from build123d import *

# Parameters (mm, degrees)
SKETCH1_R           = 19
BOSS_EXTRUDE1_DEPTH = 25
FILLET1_R           = 0.5
SKETCH3_R           = 1.55
CUT_EXTRUDE1_DEPTH  = 26.0000001
SKETCH4_R           = 6.58897104
CUT_EXTRUDE2_DEPTH  = 26.0000001
CIRPATTERN1_COUNT   = 4


with BuildPart() as part:
    # Sketch1 → Boss-Extrude1 (new body)
    with BuildSketch(Plane.XY):
        Circle(SKETCH1_R)
    extrude(amount=BOSS_EXTRUDE1_DEPTH)

    # Sketch2 → Cut-Revolve1 (revolve, cut)
    with BuildSketch(Plane(origin=(0, 0, 0), x_dir=(0, 0, -1), z_dir=(1, 0, 0))):
        with BuildLine():
            Line((-24, 19), (-21.5, 19))
            ThreePointArc((-21.5, 19), (-22.75, 18.5), (-24, 19))
        make_face()
        with BuildLine():
            Line((-3.5, 19), (-1, 19))
            ThreePointArc((-1, 19), (-2.25, 18.7), (-3.5, 19))
        make_face()
    revolve(axis=Axis((0, 0, 8.4), (0, 0, -1)), mode=Mode.SUBTRACT)

    # Fillet1
    fillet1_edges = [part.edges().sort_by_distance(p)[0] for p in [
        (-19, 0, 0),
        (-19, 0, 25),
    ]]
    fillet(fillet1_edges, radius=FILLET1_R)

    # Sketch3 → Cut-Extrude1 (cut, through all)
    with BuildSketch(Plane.XY.offset(25)):
        Circle(SKETCH3_R)
    extrude(amount=-CUT_EXTRUDE1_DEPTH, mode=Mode.SUBTRACT)

    # Sketch4 → Cut-Extrude2 (cut, through all)
    with BuildSketch(Plane.XY.offset(25)):
        with Locations((0, 10.60646011)):
            Circle(SKETCH4_R)
    cut_extrude2 = extrude(amount=-CUT_EXTRUDE2_DEPTH, mode=Mode.SUBTRACT)

    # CirPattern1: Cut-Extrude2 ×4 about axis
    cirpattern1_axis = Axis((0, 0, 0), (0, 0, 1))
    for i in range(1, CIRPATTERN1_COUNT):
        add(cut_extrude2.rotate(cirpattern1_axis, i * 360 / CIRPATTERN1_COUNT), mode=Mode.SUBTRACT)


solid = part.part
The listing builds one solid part. Answer for the finished solid, in the listing's coordinates (mm). Round coordinates to 2 decimals unless told otherwise and drop trailing zeros. Loops run counter-clockwise (first coordinate to the right, second up) from the corner with the lowest first, then second, coordinate; pieces in that order, holes last. Notation, with made-up numbers: M -33.75,58.25 L -7.75,58.25 A20 ccw -7.75,73.25 Z; hole C -5,-0.75 d4. An arc over 180 degrees is marked long. Write each question's results on one line, items separated by ' | '. Start each with the question number.
1) Find section A-A on x = 0. Count the separate pieces of the cut face and the enclosed holes in it, plus the area to 3 significant figures.
2) Straight lines are drawn through the part: probe 1 along Y at (x, z) = (5, 18.5); probe 2 along X at (y, z) = (6, 13); probe 3 along Y at (x, z) = (5.5, 16). For each, find the intervals that lie inside material, in ascending order.
3) Find section C-C on z = 10.25. Write down the section's boundary in (x, y).
4) Each of these flat-tipped pins is pushed along its axis until it touches: pin 1 (1 mm diameter, centred on y = -12.5, z = 7.5, fed in from +X); pin 2 (8 mm diameter, centred on x = -8, z = 13.5, fed in from +Y); pin 3 (6 mm diameter, centred on x = 15, z = 13.5, fed in from +Y). Where does it stop, or does it pass through?
5) Determine the mould class of faces 1 (the cylindrical face through (-0.86, 17.14, 12.68)), 2 (the cylindrical face through (18.12, 5.71, 24.25)), 3 (the flat face through (-0.26, -3.85, 25)) for opening direction X: pulls with the +X half, pulls with the -X half, needs draft (parallel to the pull), parting line crosses it, or undercut.
Final values:
1) separate pieces: 4 | enclosed holes: 0 | area: 211 mm²
2) probe 1: -18.33 to -14.9, -6.32 to -3.46, 3.46 to 6.32, 14.9 to 18.33 | probe 2: -18.03 to -13.33, -7.88 to -4.71, 4.71 to 7.88, 13.33 to 18.03 | probe 3: -18.19 to -14.23, -6.98 to -4.16, 4.16 to 6.98, 14.23 to 18.19
3) outline: C 0,0 d38; hole C -10.61,0 d13.18; hole C 0,-10.61 d13.18; hole C 0,10.61 d13.18; hole C 0,0 d3.1; hole C 10.61,0 d13.18
4) pin 1: x = 14.73 | pin 2: y = 18.57 | pin 3: y = 14.73
5) face 1: undercut | face 2: parting line crosses it | face 3: needs draft
